Read the model definition and answer for the solid it produces. Units are mm, in the model's axes. A direction names the side the tool comes from. Coordinates: 2 decimals unless noted, no trailing zeros. Write each loop counter-clockwise with the first axis right and the second up, starting at its lowest first coordinate (ties: lowest second). Pieces come first, ordered by that corner, then holes. Notation, with made-up numbers: (79, 66) -> (130, 66) arc R20 ccw to (130, 77) -> close; hole circle Ø6 at (86.25, 65.25). An arc over 180 degrees is marked (long way). One line per item, written item: value. Start each with the question number.
1. Find section D-D, the plane z = 13. Write down the section's boundary in (x, y), and give its area (3 significant figures).
2. Find section C-C, the plane y = -4. Write down the section's boundary in (x, z), and give its area (3 significant figures).
3. Find section B-B, the plane x = -2. Write down the section's boundary in (y, z), and give its area (3 significant figures).
4. Consider line 1 along Y through (x, z) = (-3, 64.5); line 2 along X through (y, z) = (-4.5, 4.5); line 3 along X through (y, z) = (29, 57). Determine where each line is inside the solid, lowest interval first.
5. Given P1, Ø11.5, axis at x = -8.71, z = 57.15, coming from the -Y side, flat-ended and moving along its own axis, determine where the tip first touches the part or whether it passes through.
6. Find section A-A, the plane z = 57.15. Write down the section's boundary in (x, y).
7. For faces 4 (the flat face through (-18, 5, 69.85)), 5 (the flat face through (-7, 28.725, 34)), determine the directions among +Z, -Z, +X, -X, +Y, -Y from which every point of the face is accessible in a straight line to the end or side of a thin tool.
8. For a pull along X with two mould halves and no side action, classify faces 1 (the flat face through (5.411, 6, 34)), 2 (the flat face through (-7, 31.9, 34)), 3 (the cylindrical face through (-8.484, 30.335, 52.113)) as pulls with the +X half, pulls with the -X half, needs draft (parallel to the pull), parting line crosses it, or undercut.
```python
from build123d import *

# Parameters (mm, degrees)
SKETCH1_W           = 25.4
SKETCH1_H           = 50.8
SKETCH1_W_2         = 19.05
SKETCH1_H_2         = 44.45
BOSS_EXTRUDE1_DEPTH = 69.85
CUT_EXTRUDE2_REACH  = 90.652
SKETCH4_R           = 5.0419


with BuildPart() as part:
    # Sketch1 → Boss-Extrude1 (new body)
    with BuildSketch(Plane.XY):
        with Locations((-7.289349112, 6.500295858)):
            Rectangle(SKETCH1_W, SKETCH1_H)
        with Locations((-7.289349112, 6.500295858)):
            Rectangle(SKETCH1_W_2, SKETCH1_H_2, mode=Mode.SUBTRACT)
    extrude(amount=BOSS_EXTRUDE1_DEPTH)

    # Cut-Extrude2: up to this face of the body (flat: up to its plane)
    cut_extrude2_end = Plane(part.part.faces().sort_by_distance((-7.289349112, -18.899704142, 34.925))[0])
    # Sketch4 → Cut-Extrude2 (cut, up to the picked face)
    with BuildSketch(Plane(origin=(0, 31.900295858, 0), x_dir=(1, 0, 0), z_dir=(0, 1, 0)), mode=Mode.PRIVATE) as cut_extrude2_sk1:
        with Locations(Location((-8.705288844, -57.15, 0), (0, 0, 270))):
            Circle(SKETCH4_R)
    cut_extrude2_tool1 = split(extrude(cut_extrude2_sk1.sketch, amount=-CUT_EXTRUDE2_REACH, mode=Mode.PRIVATE), bisect_by=cut_extrude2_end, keep=Keep.BOTH, mode=Mode.PRIVATE)
    add(cut_extrude2_tool1.solids().sort_by(Axis((-8.705289, 31.900296, 57.15), (0, -1, 0)))[0], mode=Mode.SUBTRACT)


solid = part.part
```
Answer block:
1. outline: (-19.99, -18.9) -> (5.41, -18.9) -> (5.41, 31.9) -> (-19.99, 31.9) -> close; hole (-16.81, -15.72) -> (2.24, -15.72) -> (2.24, 28.73) -> (-16.81, 28.73) -> close
1. area: 444 mm2
2. outline: (-19.99, 0) -> (-16.81, 0) -> (-16.81, 69.85) -> (-19.99, 69.85) -> close; (2.24, 0) -> (5.41, 0) -> (5.41, 69.85) -> (2.24, 69.85) -> close
2. area: 444 mm2
3. outline: (-18.9, 0) -> (-15.72, 0) -> (-15.72, 69.85) -> (-18.9, 69.85) -> close; (28.73, 0) -> (31.9, 0) -> (31.9, 69.85) -> (28.73, 69.85) -> close
3. area: 444 mm2
4. line 1: y = -18.9 to -15.72, 28.73 to 31.9
4. line 2: x = -19.99 to -16.81, 2.24 to 5.41
4. line 3: x = -19.99 to -13.74, -3.67 to 5.41
5. P1: stops at y = -18.9
6. outline: (-19.99, -18.9) -> (-13.75, -18.9) -> (-13.75, -15.72) -> (-16.81, -15.72) -> (-16.81, 28.73) -> (-13.75, 28.73) -> (-13.75, 31.9) -> (-19.99, 31.9) -> close; (-3.66, -18.9) -> (5.41, -18.9) -> (5.41, 31.9) -> (-3.66, 31.9) -> (-3.66, 28.73) -> (2.24, 28.73) -> (2.24, -15.72) -> (-3.66, -15.72) -> close
7. face 4: +Z, +X, -X, +Y, -Y
7. face 5: +Z, -Z
8. face 1: pulls with the +X half
8. face 2: needs draft
8. face 3: undercut
